The model under review builds one solid part; all positions refer to its coordinate system, in mm. A direction names the side the tool comes from. Coordinates: 2 decimals unless noted, no trailing zeros. Write each loop counter-clockwise with the first axis right and the second up, starting at its lowest first coordinate (ties: lowest second). Pieces come first, ordered by that corner, then holes. Notation, with made-up numbers: (-20, 15.25) - (3, 15.25) arc R32 ccw to (3, 47.25) - close; hole circle Ø5 at (74.25, 65.5). An arc over 180 degrees is marked (long way). Use one line per item in the form item = value. Start each with the question number.
Autodesk Inventor part; units mm, degrees
ref_plane "YZ Plane" through (0, 0, 0) normal (1, 0, 0) x (0, 1, 0)
ref_plane "XZ Plane" through (0, 0, 0) normal (0, 1, 0) x (-1, 0, 0)
ref_plane "XY Plane" through (0, 0, 0) normal (0, 0, 1) x (1, 0, 0)
sketch "Sketch1" plane through (0, 0, 0) normal (0, 0, 1) x (1, 0, 0)
  line L0 (0, 0) -> (0, -25.4)
  line L1 (0, -25.4) -> (-2.3749, -25.4)
  line L2 (-4.7625, -23.0124) -> (-4.7625, -7.9375)
  line L3 (-7.9375, -4.7625) -> (-23.0124, -4.7625)
  line L4 (-25.4, -2.3749) -> (-25.4, 0)
  line L5 (-25.4, 0) -> (0, 0)
  arc A0 (-4.7625, -7.9375) -> (-7.9375, -4.7625) centre (-7.9375, -7.9375) ccw
  arc A1 (-25.4, -2.3749) -> (-23.0124, -4.7625) centre (-23.0124, -2.3749) ccw
  arc A2 (-4.7625, -23.0124) -> (-2.3749, -25.4) centre (-2.3749, -23.0124) ccw
  dimension "d2" = 25.4
  dimension "d3" = 4.7625
  dimension "d4" = 3.175
  dimension "d5" = 2.3876
extrude "Extrusion1" add sketch "Sketch1" along normal blind 50.8
properties part number "GE-12026-06"
1. For P1, Ø12, axis at x = -14.5, z = 37.5, coming from the -Y side; P2, Ø1.5, axis at y = -7.5, z = 19, coming from the +X side; P3, Ø7.5, axis at y = -16.5, z = 23, coming from the -X side; P4, Ø4, axis at y = -5, z = 24.5, coming from the -X side, all flat-tipped, find the tip position at first contact; note any pin that passes through.
2. For faces 1 (the flat face through (-25.4, -1, 25)), 2 (the flat face through (-15, -4.762, 25)), list the 3-axis set-ups (+Z, -Z, +X, -X, +Y, -Y) from which the entire face can be reached by the end or side of a thin tool; tool diameter is ignored.
3. Take a section at B-B (x = -19.25). State the section outline as (y, z) points.
4. For L1, parallel to Y at x = -13.5, z = 44; L2, parallel to Y at x = -4.5, z = 5, list the stretches that pass through material, from the lowest coordinate up.
Returned:
q1.P1 = -4.76
q1.P2 = 0
q1.P3 = -4.76
q1.P4 = -25.32
q2.face_1 = +Z, -Z, -X, +Y, -Y
q2.face_2 = +Z, -Z, -X, -Y
q3.outline = (-4.76, 0) - (0, 0) - (0, 50.8) - (-4.76, 50.8) - close
q4.L1 = -4.76 to 0
q4.L2 = -24.1 to 0
